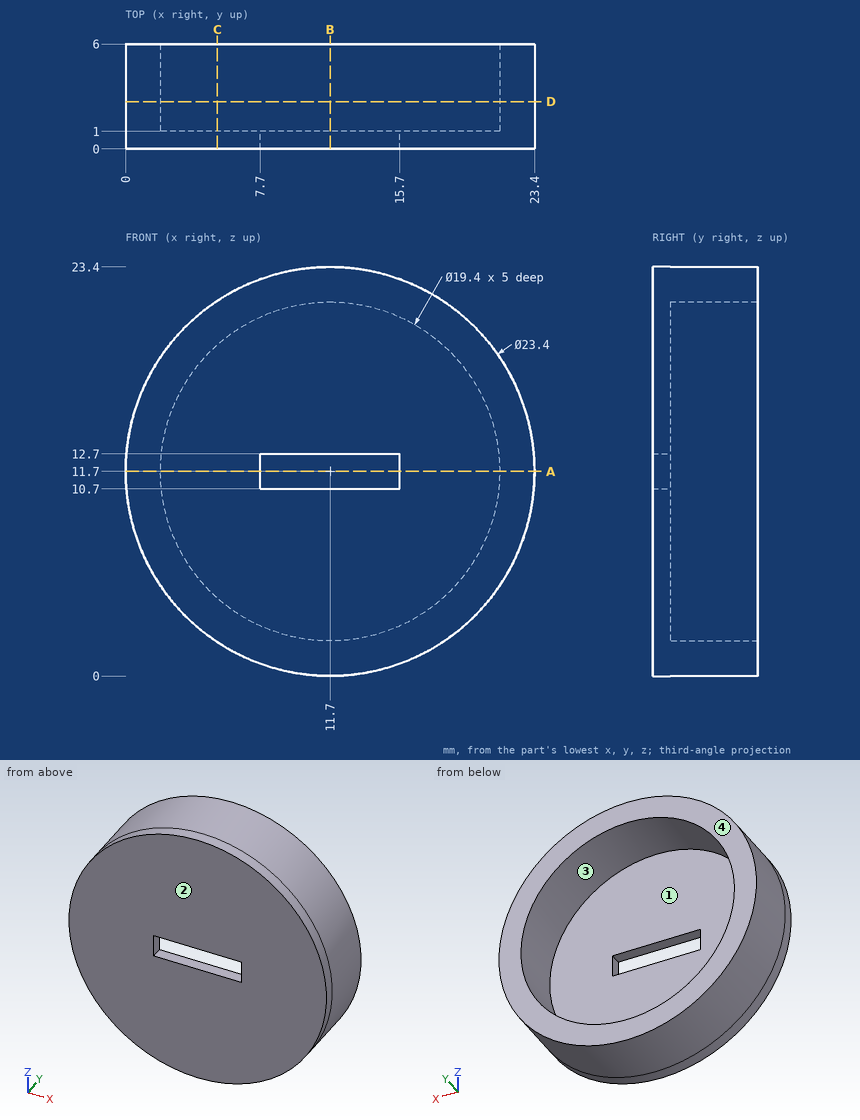
The figure shows three views and two pictorial views of one solid part (mm, origin at its lowest corner). Answer the questions. A direction names the side the tool comes from. Give positions to 0.01 mm unless a question says otherwise; leave off trailing zeros. Order: outer loops, then holes, each group sorted by start corner. A loop starts at its lowest first (then second) coordinate and runs counter-clockwise, first axis right, second up. Notation, with made-up numbers: M 16.25,-40 L 29.25,-40 A22 cw 29.25,-10 Z; hole C 54.5,74 d8. An arc over 180 degrees is marked long. Return JSON: item names as keys, results as strings.
Q1. Find section C-C, the plane x = 5.25. Write down the section's boundary in (y, z).
Answer below:
{"outline": "M 0,1.94 L 6,1.94 L 6,4.46 L 1,4.46 L 1,18.94 L 6,18.94 L 6,21.46 L 0,21.46 Z"}
Q2. Find section D-D, the plane y = 2.7. Write down the section's boundary in (x, z).
Answer below:
{"outline": "C 11.7,11.7 d23.4; hole C 11.7,11.7 d19.4"}
Q3. Which of the six approach directions +Z, -Z, +X, -X, +Y, -Y give full straight-line access (tool end or side, diameter ignored) to the marked faces 1 and 2?
Answer below:
{"face 1": "+Y", "face 2": "+Z, -Z, +X, -X, -Y"}
Q4. Find the intervals of material crossed by line 1 along X through (y, z) = (2.6, 11.7); line 2 along Y through (x, z) = (9, 20.5); line 3 along Z through (x, y) = (9.5, 2.8), in increasing order. Write a range as [from, to].
Answer below:
{"line 1": "x = [0, 2], [21.4, 23.4]", "line 2": "y = [0, 1]", "line 3": "z = [0.21, 2.25], [21.15, 23.19]"}
Q5. The mould has two halves that part along Z. Classify the marked faces 3 and 4: pulls with the +Z half, pulls with the -Z half, needs draft (parallel to the pull), parting line crosses it, or undercut.
Answer below:
{"face 3": "undercut", "face 4": "needs draft"}
Q6. Each of these flat-tipped pins is pushed along its axis until it touches: pin 1 (8 mm diameter, centred on x = 13.5, z = 12.5, fed in from +Y); pin 2 (0.5 mm diameter, centred on x = 11, y = 0.5, fed in from -Z); pin 3 (1.1 mm diameter, centred on x = 10.5, y = 0.5, fed in from +Z). Where does it stop, or does it pass through?
Answer below:
{"pin 1": "stops at y = 1", "pin 2": "stops at z = 0.01", "pin 3": "stops at z = 23.38"}
Q7. Find section B-B, the plane x = 11.7. Write down the section's boundary in (y, z), and give its area (3 significant figures).
Answer below:
{"outline": "M 0,0 L 6,0 L 6,2 L 1,2 L 1,10.7 L 0,10.7 Z; M 0,12.7 L 1,12.7 L 1,21.4 L 6,21.4 L 6,23.4 L 0,23.4 Z", "area": "41.4 mm^2"}
Q8. Find section A-A, the plane z = 11.7. Write down the section's boundary in (x, y), and give its area (3 significant figures).
Answer below:
{"outline": "M 0,0 L 7.7,0 L 7.7,1 L 2,1 L 2,6 L 0,6 Z; M 15.7,0 L 23.4,0 L 23.4,6 L 21.4,6 L 21.4,1 L 15.7,1 Z", "area": "35.4 mm^2"}
